Geometry check sheet. Reference: the model listing, model coordinates, mm. Face numbers are marked on the shaded views. A direction names the side the tool comes from. Round coordinates to 2 decimals unless told otherwise and drop trailing zeros. Write each loop counter-clockwise with the first axis right and the second up, starting at its lowest first coordinate (ties: lowest second). Pieces come first, ordered by that corner, then holes. Notation, with made-up numbers: M 88.5,18.25 L 147.5,18.25 A8 cw 147.5,29.25 Z; hole C 31.5,-30 d8. An arc over 180 degrees is marked long. Put each result on its own line as item: value. Start each with the question number.
(1) Section check C-C on y = 653. Record the cut outline in (x, z).
(2) Material ranges on probe 1 along X at (y, z) = (-653.5, -4); probe 2 along Y at (x, z) = (-48, 32.5); probe 3 along Z at (x, y) = (16.5, 36.5), recorded low to high.
(3) Tool access check on the marked faces 1 and 2. Record the directions out of +Z, -Z, +X, -X, +Y, -Y that give a thin tool (end or side, any length) a straight path to the whole face; none if there is none.
(4) Section check A-A on z = 33. Record the cut outline in (x, y), then the cut area to 3 significant figures.
(5) Section check B-B on x = 16.5. Record the cut outline in (y, z), then the cut area to 3 significant figures.
(6) Gauge pin test, flat ends, axial feed: pin 1 (1.5 mm diameter, centred on x = -3.5, y = -662, fed in from +Z); pin 2 (12 mm diameter, centred on x = -40.5, y = 532.5, fed in from -Z); pin 3 (1 mm diameter, centred on y = -221, z = -48, fed in from -X). Record the tip position at first contact, or that the pin passes through.
from build123d import *

# Parameters (mm, degrees)
F0_R     = 62.5
F1_DEPTH = 1050
F2_R     = 62.5
F2_R_2   = 60
F3_DEPTH = 240
F2_R_3   = 55
F4_DEPTH = 160


with BuildPart() as f1:
    # F0 (on Front) → F1 (new body, symmetric)
    with BuildSketch(Plane.XZ):
        Circle(F0_R)
    extrude(amount=F1_DEPTH, both=True)

    # F2 (on face) → F3 (cut)
    with BuildSketch(Plane(origin=(0, 1050, 0), x_dir=(-1, 0, 0), z_dir=(0, 1, 0))):
        Circle(F2_R)
        Circle(F2_R_2, mode=Mode.SUBTRACT)
    extrude(amount=-F3_DEPTH, mode=Mode.SUBTRACT)

    # F2 (on face) → F4 (cut)
    with BuildSketch(Plane(origin=(0, 1050, 0), x_dir=(-1, 0, 0), z_dir=(0, 1, 0))):
        Circle(F2_R_2)
        Circle(F2_R_3, mode=Mode.SUBTRACT)
    extrude(amount=-F4_DEPTH, mode=Mode.SUBTRACT)


solid = f1.part
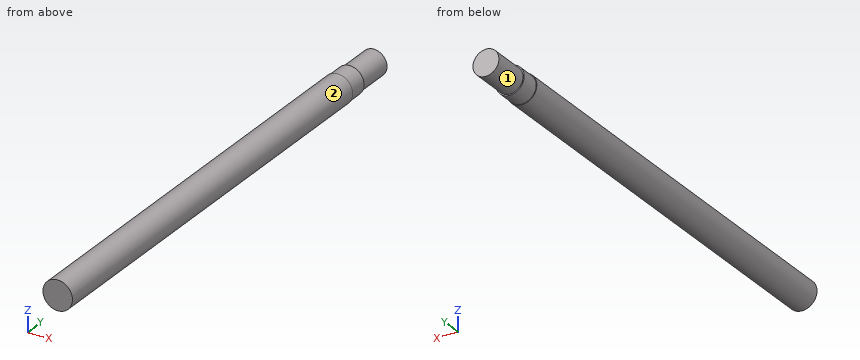
Answers follow:
1. outline: C 0,0 d125
2. probe 1: x = -62.37 to 62.37
2. probe 2: y = -1050 to 890
2. probe 3: z = -60.28 to 60.28
3. face 1: +Y
3. face 2: +Y, -Y
4. outline: M -53.08,-1050 L 53.08,-1050 L 53.08,810 L 50.11,810 L 50.11,890 L 44,890 L 44,1050 L -44,1050 L -44,890 L -50.11,890 L -50.11,810 L -53.08,810 Z
4. area: 220,000 mm^2
5. outline: M -1050,-60.28 L 810,-60.28 L 810,-57.69 L 890,-57.69 L 890,-52.47 L 1050,-52.47 L 1050,52.47 L 890,52.47 L 890,57.69 L 810,57.69 L 810,60.28 L -1050,60.28 Z
5. area: 250,000 mm^2
6. pin 1: stops at z = 62.44
6. pin 2: stops at z = -52.12
6. pin 3: stops at x = -40.62
